Geometry check sheet. Reference: the model listing, model coordinates, mm. Round coordinates to 2 decimals unless told otherwise and drop trailing zeros. Order: outer loops, then holes, each group sorted by start corner. A loop starts at its lowest first (then second) coordinate and runs counter-clockwise, first axis right, second up. Notation, with made-up numbers: (-32, -4) -> (-24, -4) arc R23 ccw to (-24, 17) -> close; hole circle Ø1 at (11, 3). An arc over 180 degrees is marked (long way). Answer as a JSON object with one key per item and string values. Group by question number.
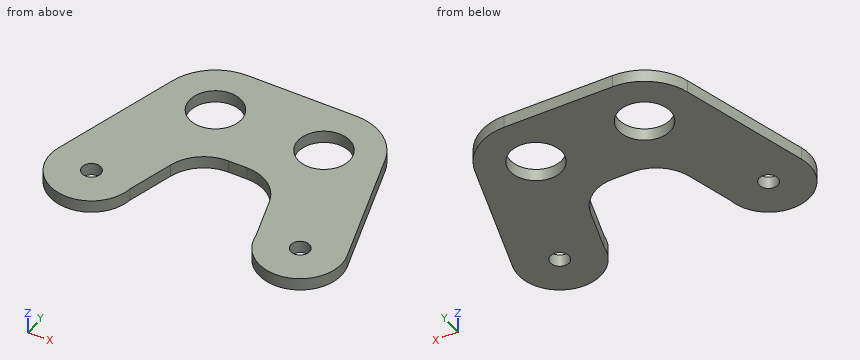
from build123d import *

# Parameters (mm, degrees)
ESQUISSE1_R          = 10
ESQUISSE1_R_2        = 2.25
BOSS_EXTRU_1_DEPTH   = 3
BOSS_EXTRU_1_2_DEPTH = 3
ESQUISSE1_R_3        = 6.25
BOSS_EXTRU_1_3_DEPTH = 3
BOSS_EXTRU_2_DEPTH   = 3
CONG_1_R             = 10


with BuildPart() as part:
    # Esquisse1 → Boss.-Extru.1 (new body)
    with BuildSketch(Plane.XY):
        Circle(ESQUISSE1_R)
        Circle(ESQUISSE1_R_2, mode=Mode.SUBTRACT)
    extrude(amount=BOSS_EXTRU_1_DEPTH)



with BuildPart() as body_2:
    # Esquisse1 → Boss.-Extru.1 2 (new body)
    with BuildSketch(Plane.XY):
        with Locations((50, 0)):
            Circle(ESQUISSE1_R)
        with Locations((50, 0)):
            Circle(ESQUISSE1_R_2, mode=Mode.SUBTRACT)
    extrude(amount=BOSS_EXTRU_1_2_DEPTH)


with BuildPart() as body_3:
    # Esquisse1 → Boss.-Extru.1 3 (new body)
    with BuildSketch(Plane.XY):
        with BuildLine():
            Line((12, 43), (38, 43))
            ThreePointArc((38, 43), (51, 30), (38, 17))
            Line((38, 17), (12, 17))
            ThreePointArc((12, 17), (-1, 30), (12, 43))
        make_face()
        with Locations((12, 30)):
            Circle(ESQUISSE1_R_3, mode=Mode.SUBTRACT)
        with Locations((38, 30)):
            Circle(ESQUISSE1_R_3, mode=Mode.SUBTRACT)
    extrude(amount=BOSS_EXTRU_1_3_DEPTH)


with BuildPart() as part_1:
    add(part.part)

    add(body_2.part)  # Boss.-Extru.2 merges body 2

    add(body_3.part)  # Boss.-Extru.2 merges body 3
    # Esquisse2 → Boss.-Extru.2 (add)
    with BuildSketch(Plane.XY.offset(3)):
        with BuildLine():
            ThreePointArc((12, 17), (1.585468462, 22.219413078), (-0.46633352, 33.686533408))
            Line((-0.46633352, 33.686533408), (-9.589487323, 2.835794929))
            ThreePointArc((-9.589487323, 2.835794929), (2.00193965, 9.797562842), (9.933272577, -1.153297843))
            Line((9.933272577, -1.153297843), (15.301550175, 17))
            Line((15.301550175, 17), (12, 17))
        make_face()
        with BuildLine():
            Line((38, 17), (34.698449825, 17))
            Line((34.698449825, 17), (40.066727423, -1.153297843))
            ThreePointArc((40.066727423, -1.153297843), (47.99806035, 9.797562842), (59.589487323, 2.835794929))
            Line((59.589487323, 2.835794929), (50.46633352, 33.686533408))
            ThreePointArc((50.46633352, 33.686533408), (48.414531538, 22.219413078), (38, 17))
        make_face()
    extrude(amount=-BOSS_EXTRU_2_DEPTH)

    # Congé1
    cong_1_edges = [part_1.edges().sort_by_distance(p)[0] for p in [
        (15.301550175, 17, 1.5),
        (34.698449825, 17, 1.5),
    ]]
    fillet(cong_1_edges, radius=CONG_1_R)


solid = part_1.part
Item 1: Sectioned sample at B-B, the plane z = 2.45. Enter the section's corners in (x, y).
Item 2: Thickness scan on L1, parallel to X at y = 33, z = 0.9; L2, parallel to X at y = 34, z = 0.6; L3, parallel to X at y = 8, z = 1.25. Record the ranges inside material, lowest first.
Item 3: Sectioned sample at D-D, the plane y = 8.5. Enter the section's corners in (x, z), then the cut area to 3 significant figures.
Item 4: Sectioned sample at A-A, the plane y = 31. Enter the section's corners in (x, z).
Item 5: Depth check by flat-ended pin: pin 1 Ø1 at (x, z) = (6.5, 1.5) entering from +Y. Enter the tip coordinate at first touch or a pass-through.
Item 6: Sectioned sample at C-C, the plane x = 1. Enter the section's corners in (y, z), then the cut area to 3 significant figures.
Result:
{
 "1": {"outline": "(-9.59, 2.84) arc R10 ccw (long way) to (9.93, -1.15) -> (13.18, 9.84) arc R10 cw to (22.77, 17) -> (27.23, 17) arc R10 cw to (36.82, 9.84) -> (40.07, -1.15) arc R10 ccw (long way) to (59.59, 2.84) -> (50.47, 33.69) arc R13 ccw to (38, 43) -> (12, 43) arc R13 ccw to (-0.47, 33.69) -> close; hole circle Ø4.5 at (0, 0); hole circle Ø12.5 at (12, 30); hole circle Ø12.5 at (38, 30); hole circle Ø4.5 at (50, 0)"},
 "2": {"L1": "x = -0.67 to 6.52, 17.48 to 32.52, 43.48 to 50.67", "L2": "x = -0.37 to 7.2, 16.8 to 33.2, 42.8 to 50.37", "L3": "x = -8.06 to 12.64, 37.36 to 58.06"},
 "3": {"outline": "(-7.91, 0) -> (12.79, 0) -> (12.79, 3) -> (-7.91, 3) -> close; (37.21, 0) -> (57.91, 0) -> (57.91, 3) -> (37.21, 3) -> close", "area": "124 mm2"},
 "4": {"outline": "(-1.26, 0) -> (5.83, 0) -> (5.83, 3) -> (-1.26, 3) -> close; (18.17, 0) -> (31.83, 0) -> (31.83, 3) -> (18.17, 3) -> close; (44.17, 0) -> (51.26, 0) -> (51.26, 3) -> (44.17, 3) -> close"},
 "5": {"pin 1": "stops at y = 42"},
 "6": {"outline": "(-9.95, 0) -> (-2.02, 0) -> (-2.02, 3) -> (-9.95, 3) -> close; (2.02, 0) -> (36.93, 0) -> (36.93, 3) -> (2.02, 3) -> close", "area": "129 mm2"}
}
